from build123d import *

# Parameters (mm, degrees)
SKETCH_R           = 30
SKETCH_R_2         = 25
PAD003_DEPTH       = 6
PAD003_DEPTH_BACK  = 15
SKETCH001_R        = 5
PAD004_DEPTH       = 30
POLARPATTERN_COUNT = 4
SKETCH003_R        = 25
SKETCH003_R_2      = 20
PAD_DEPTH          = 10
SKETCH004_R        = 5
SKETCH004_R_2      = 2.5
PAD006_DEPTH       = 4
PAD006_DEPTH_BACK  = 30
SKETCH005_R        = 2.5
POCKET_DEPTH       = 30.001
POCKET_DEPTH_BACK  = 30.001


with BuildPart() as part:
    # Sketch → Pad003 (new body, two sides)
    with BuildSketch(Plane.XY) as pad003_sk:
        Circle(SKETCH_R)
        Circle(SKETCH_R_2, mode=Mode.SUBTRACT)
    extrude(amount=PAD003_DEPTH)
    extrude(pad003_sk.sketch, amount=-PAD003_DEPTH_BACK)

    # Sketch001 → Pad004 (join)
    with BuildSketch(Plane.XY):
        with Locations((0, 22)):
            Circle(SKETCH001_R)
    pad004 = extrude(amount=PAD004_DEPTH)

    # PolarPattern: Pad004 ×4 about axis
    polarpattern_axis = Axis((0, 0, 0), (0, 0, 1))
    for i in range(1, POLARPATTERN_COUNT):
        add(pad004.rotate(polarpattern_axis, i * 360 / POLARPATTERN_COUNT))

    # Sketch003 → Pad (join)
    with BuildSketch(Plane.XY):
        Circle(SKETCH003_R)
        Circle(SKETCH003_R_2, mode=Mode.SUBTRACT)
    extrude(amount=PAD_DEPTH)

    # Sketch004 → Pad006 (join, two sides)
    with BuildSketch(Plane.XY) as pad006_sk:
        with Locations((17.614592, 17.594242)):
            Circle(SKETCH004_R)
        with Locations((17.66179, 17.660632)):
            Circle(SKETCH004_R_2, mode=Mode.SUBTRACT)
    extrude(amount=PAD006_DEPTH)
    extrude(pad006_sk.sketch, amount=-PAD006_DEPTH_BACK)

    # Sketch005 → Pocket (cut, two sides)
    with BuildSketch(Plane.XY) as pocket_sk:
        with Locations((17.681431, 17.632393)):
            Circle(SKETCH005_R)
    extrude(amount=-POCKET_DEPTH, mode=Mode.SUBTRACT)
    extrude(pocket_sk.sketch, amount=POCKET_DEPTH_BACK, mode=Mode.SUBTRACT)


solid = part.part
The listing builds one solid part. Answer for the finished solid, in the listing's coordinates (mm). A direction names the side the tool comes from. Give positions to 0.01 mm unless a question says otherwise; leave off trailing zeros. Order: outer loops, then holes, each group sorted by start corner. A loop starts at its lowest first (then second) coordinate and runs counter-clockwise, first axis right, second up. Notation, with made-up numbers: (76, 85.25) - (98, 85.25) arc R24 cw to (98, 111.25) - close; hole circle Ø11 at (-19.75, 1). An arc over 180 degrees is marked (long way). One line per item, written item: value. Start each with the question number.
1) Find the intervals of material crossed by L1, parallel to Y at x = 0, z = -4.5; L2, parallel to Z at x = -23, y = -8; L3, parallel to Z at x = 14, y = 23, in increasing order.
2) Given pin 1 Ø10 at (x, y) = (21.5, 19) entering from +Z; pin 2 Ø5 at (x, z) = (-6.5, 7) entering from +Y; pin 3 Ø22.5 at (x, y) = (-12.5, -9.5) entering from +Z; pin 4 Ø5 at (y, z) = (3.5, 14.5) entering from -X, each flat-ended and moving along its own axis, determine where each tip first touches the part or whether it passes through.
3) A cutting plane is placed at C-C on z = 19. Give the vertices of the cut face in (x, y), then the cut area to 3 significant figures.
4) The mould has two halves that part along X. Classify faces 1 (the face through (14.03, -14.254, 4.93)), 2 (the face through (22, 0, 30)), 3 (the face through (17.525, -17.829, 7.972)), 4 (the face through (-17.829, -17.525, 7.972)): released by +X, released by -X, zero draft, split by the parting line, or undercut.
5) A cutting plane is placed at D-D on z = -3. State how many separate pieces and enclosed holes the cut face has, then the cut area to 3 significant figures.
6) A tool of negligible diameter and unlimited length cuts with its end or side. For faces 5 (the face through (-17.525, 17.829, 7.972)), 6 (the face through (1.08, -17.12, 18.12)), 7 (the face through (10.47, 22.7, 7.97)), 8 (the face through (-14.254, -14.03, 4.93)), from which of +Z, -Z, +X, -X, +Y, -Y can it reach the whole face along a straight path? Write none if from no direction.
7) A cutting plane is placed at A-A on x = 0. Give the vertices of the cut face in (y, z).
Answer sheet:
1. L1: y = -30 to -25, 25 to 30
1. L2: z = 0 to 10
1. L3: z = -15 to 6
2. pin 1: stops at z = 10
2. pin 2: stops at y = 29.7
2. pin 3: stops at z = 30
2. pin 4: stops at x = -26.9
3. outline: circle Ø10 at (-22, 0); circle Ø10 at (0, -22); circle Ø10 at (0, 22); circle Ø10 at (22, 0)
3. area: 314 mm2
4. face 1: undercut
4. face 2: zero draft
4. face 3: released by +X
4. face 4: released by -X
5. separate pieces: 1
5. enclosed holes: 2
5. area: 883 mm2
6. face 5: +Z, -X, +Y
6. face 6: +Z
6. face 7: +Z, +X, +Y
6. face 8: +Z, -Z
7. outline: (-30, -15) - (-25, -15) - (-25, 0) - (-17, 0) - (-17, 30) - (-27, 30) - (-27, 6) - (-30, 6) - close; (17, 0) - (25, 0) - (25, -15) - (30, -15) - (30, 6) - (27, 6) - (27, 30) - (17, 30) - close
